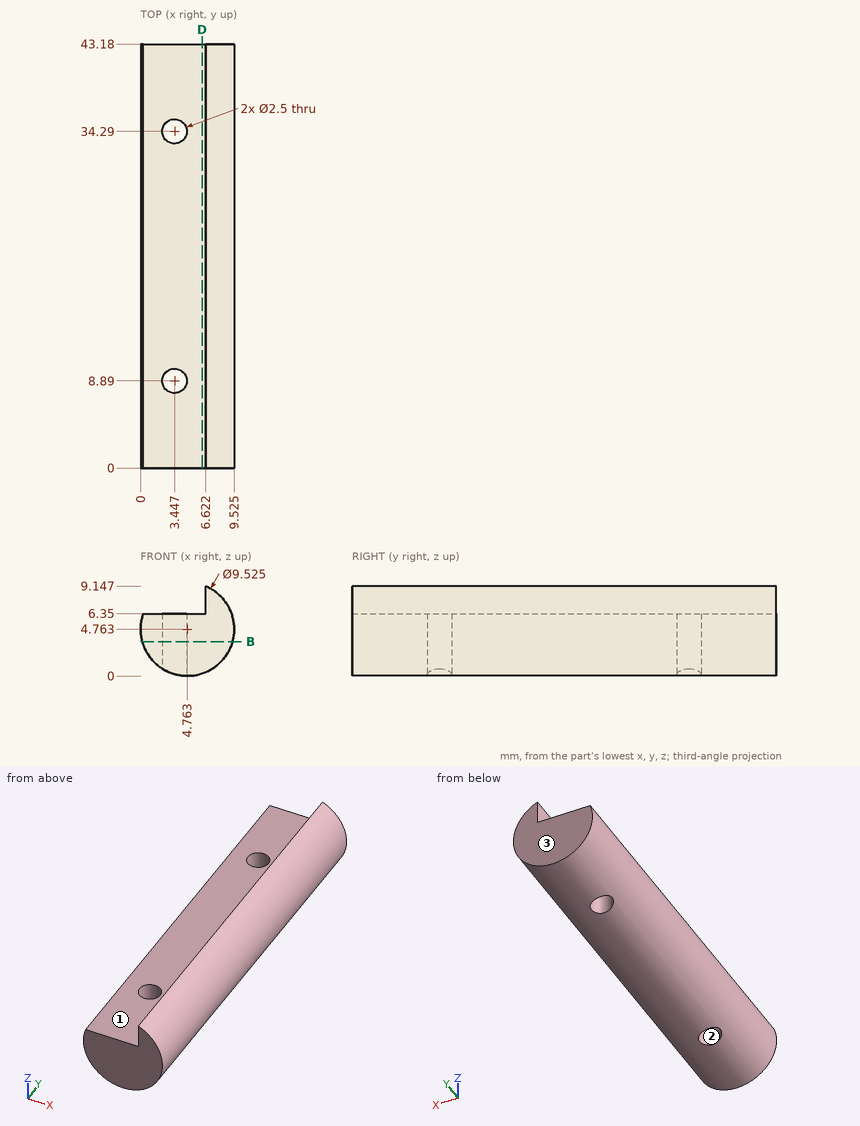
Could you check a few things on this drawing? It's one solid part, dimensions in mm from its lowest x, y, z. Give positions to 0.01 mm unless a question says otherwise; leave off trailing zeros. Write each loop counter-clockwise with the first axis right and the second up, starting at its lowest first coordinate (ties: lowest second). Pieces come first, ordered by that corner, then holes. Notation, with made-up numbers: (40.5, 53.25) -> (91.5, 53.25) arc R31 cw to (91.5, 91.25) -> close; hole circle Ø10 at (22.25, -14.5). An arc over 180 degrees is marked (long way). Write item = value, one per line.
(1) Thinking about a two-plate mould opening in Y: for the marked faces 1, 2 and 3, which applies, released by +Y, released by -Y, zero draft, split by the parting line, or undercut?
Worked out:
face_1 = zero draft
face_2 = undercut
face_3 = released by +Y
(2) Suppose I cut it at D-D on x = 6.25. Write out the boundary of the cut face in (y, z), then the cut area to 3 significant figures.
Worked out:
outline = (0, 0.24) -> (43.18, 0.24) -> (43.18, 6.35) -> (0, 6.35) -> close
area = 264 mm^2
(3) I need wall thicknesses on probe 1 along Y at (x, z) = (2.5, 5.25) (1 decimal); probe 2 along X at (y, z) = (4, 5) (1 decimal); probe 3 along Y at (x, z) = (4, 4.5). Which ranges of each line are inside material? Lowest first, please. Write a range as from..to.
Worked out:
probe_1 = 0..8.1, 9.7..33.5, 35.1..43.2
probe_2 = 0..9.5
probe_3 = 0..7.77, 10.01..33.17, 35.41..43.18
(4) I'm going to push flat-ended pins straight in: P1, Ø5, axis at x = 2, y = 23.5, coming from the +Z side; P2, Ø1, axis at y = 37.5, z = 8, coming from the +X side; P3, Ø1, axis at x = 5.5, y = 18.5, coming from the -Z side; P4, Ø5, axis at y = 8, z = 6, coming from the -X side. Where does each tip first touch, or does it pass through?
Worked out:
P1 = 6.35
P2 = 8.66
P3 = 0.01
P4 = 0
(5) Suppose I cut it at B-B on z = 3.5. Count the separate pieces of the cut face and the enclosed holes in it, then the cut area to 3 significant figures.
Worked out:
separate_pieces = 1
enclosed_holes = 2
area = 387 mm^2
